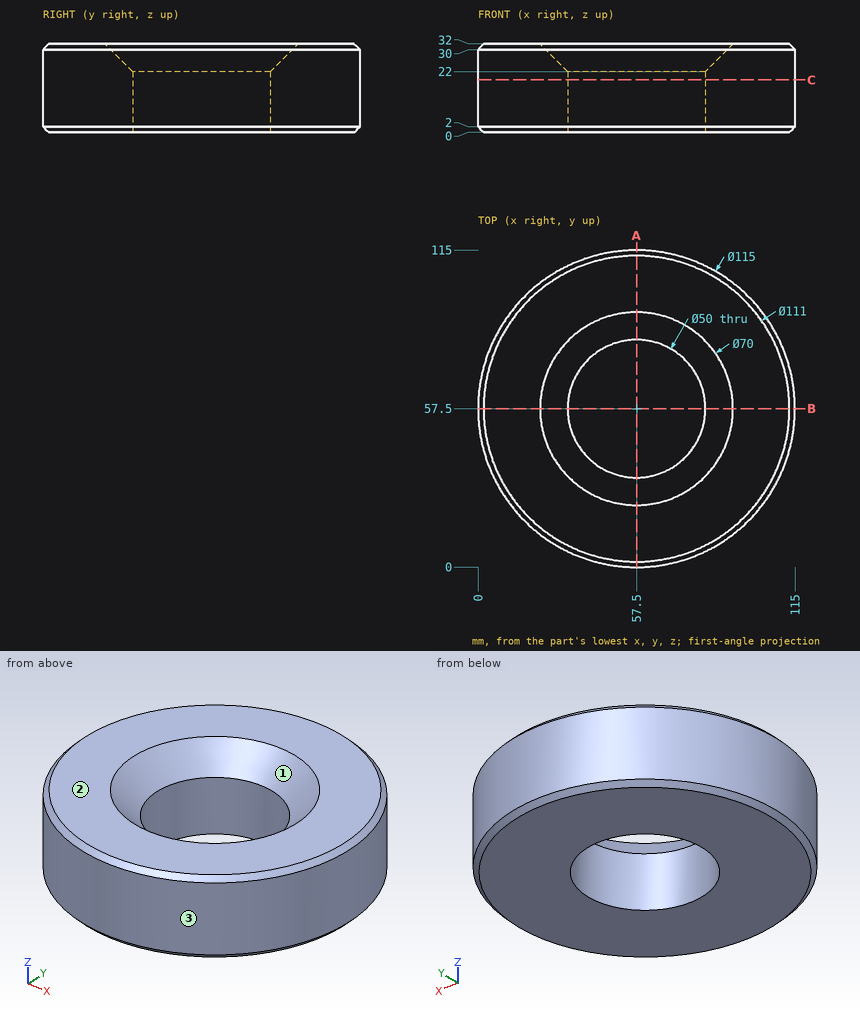
Job drawing, mm, ordinate dimensions from the low corner. One solid piece. Round coordinates to 2 decimals unless told otherwise and drop trailing zeros. Write each loop counter-clockwise with the first axis right and the second up, starting at its lowest first coordinate (ties: lowest second). Pieces come first, ordered by that corner, then holes.
1) Drill centre lines: probe 1 along Y at (x, z) = (57, 13) (3 decimals); probe 2 along X at (y, z) = (39, 13.5). Where is each one in solid material? Low to high.
2) Pin check, flat tips, straight feed: pin 1 (4 mm diameter, centred on y = 20.5, z = 12, fed in from -X); pin 2 (8 mm diameter, centred on x = 32, z = 25, fed in from -Y); pin 3 (3 mm diameter, centred on y = 95, z = 19.5, fed in from +X). Stop position of each tip, or through.
3) Mould opens along X. For the marked faces 1, 2 and 3 say: +X half, -X half, draft (parallel to the pull), parting line (faces both ways), or undercut.
4) Band-saw the part on A-A, the plane x = 57.5. List the corners of the cut face in (y, z).
5) Band-saw the part on C-C, the plane z = 19. List the corners of the cut face in (x, y), and give its area (3 significant figures).
Ans:
1. probe 1: y = 0.002 to 32.505, 82.495 to 114.998
1. probe 2: x = 3.06 to 40.68, 74.32 to 111.94
2. pin 1: stops at x = 11.88
2. pin 2: stops at y = 4.17
2. pin 3: stops at x = 102.34
3. face 1: undercut
3. face 2: draft
3. face 3: parting line
4. outline: (0, 2) - (2, 0) - (32.5, 0) - (32.5, 22) - (22.5, 32) - (2, 32) - (0, 30) - close; (82.5, 0) - (113, 0) - (115, 2) - (115, 30) - (113, 32) - (92.5, 32) - (82.5, 22) - close
5. outline: circle Ø115 at (57.5, 57.5); hole circle Ø50 at (57.5, 57.5)
5. area: 8,420 mm2
